```python
from build123d import *

# Parameters (mm, degrees)
SKETCH_1_R          = 1.6
EXTRUDE_1_DEPTH     = 3
SKETCH_2_W          = 11
SKETCH_2_H          = 38
CUT_EXTRUDE_1_DEPTH = 1
CUT_EXTRUDE_START   = -2
CUT_EXTRUDE_2_DEPTH = 2
SKETCH_4_R          = 1.6
CUT_EXTRUDE_3_DEPTH = 62.990079852
SKETCH_6_R          = 2
CUT_EXTRUDE_4_DEPTH = 1
SKETCH_7_R          = 4.1
CUT_EXTRUDE_5_DEPTH = 63.030395775
FILLET_1_R          = 1


with BuildPart() as part:
    # 草图1 → 凸台-拉伸1 (new body)
    with BuildSketch(Plane.XY):
        with BuildLine():
            Line((47.4, -34.9), (47.4, 34.9))
            ThreePointArc((47.4, 34.9), (45.935533906, 38.435533906), (42.4, 39.9))
            Line((42.4, 39.9), (21.6, 39.9))
            ThreePointArc((21.6, 39.9), (18.064466094, 38.435533906), (16.6, 34.9))
            Line((16.6, 34.9), (16.6, -34.9))
            ThreePointArc((16.6, -34.9), (18.064466094, -38.435533906), (21.6, -39.9))
            Line((21.6, -39.9), (42.4, -39.9))
            ThreePointArc((42.4, -39.9), (45.935533906, -38.435533906), (47.4, -34.9))
        make_face()
        with Locations((37.413843028, 25.79305128)):
            Circle(SKETCH_1_R, mode=Mode.SUBTRACT)
        with Locations((31.413843028, 25.79305128)):
            Circle(SKETCH_1_R, mode=Mode.SUBTRACT)
        with BuildLine():
            Line((40.513850359, -21.477641558), (40.513850359, -10.127641653))
            ThreePointArc((40.513850359, -10.127641653), (40.367403749, -9.774088262), (40.013850359, -9.627641653))
            Line((40.013850359, -9.627641653), (30.013850359, -9.627641653))
            ThreePointArc((30.013850359, -9.627641653), (29.660296968, -9.774088262), (29.513850359, -10.127641653))
            Line((29.513850359, -10.127641653), (29.513850359, -21.477641558))
            ThreePointArc((29.513850359, -21.477641558), (29.660296968, -21.831194949), (30.013850359, -21.977641558))
            Line((30.013850359, -21.977641558), (40.013850359, -21.977641558))
            ThreePointArc((40.013850359, -21.977641558), (40.367403749, -21.831194949), (40.513850359, -21.477641558))
        make_face(mode=Mode.SUBTRACT)
        with BuildLine():
            Line((40.464996896, 6.495389649), (40.464996896, -6.604609867))
            ThreePointArc((40.464996896, -6.604609867), (40.406418252, -6.746031223), (40.264996896, -6.804609867))
            Line((40.264996896, -6.804609867), (28.963873947, -6.804609867))
            ThreePointArc((28.963873947, -6.804609867), (28.822452591, -6.746031223), (28.763873947, -6.604609867))
            Line((28.763873947, -6.604609867), (28.763873947, 6.495389649))
            ThreePointArc((28.763873947, 6.495389649), (28.822452591, 6.636811005), (28.963873947, 6.695389649))
            Line((28.963873947, 6.695389649), (40.264996896, 6.695389649))
            ThreePointArc((40.264996896, 6.695389649), (40.406418252, 6.636811005), (40.464996896, 6.495389649))
        make_face(mode=Mode.SUBTRACT)
        with BuildLine():
            Line((40.513843009, 11.302412116), (40.513843009, 19.702429875))
            ThreePointArc((40.513843009, 19.702429875), (40.396685721, 19.985272588), (40.113843009, 20.102429875))
            Line((40.113843009, 20.102429875), (29.713821303, 20.102429875))
            ThreePointArc((29.713821303, 20.102429875), (29.43097859, 19.985272588), (29.313821303, 19.702429875))
            Line((29.313821303, 19.702429875), (29.313821303, 11.302412116))
            ThreePointArc((29.313821303, 11.302412116), (29.43097859, 11.019569403), (29.713821303, 10.902412116))
            Line((29.713821303, 10.902412116), (40.113843009, 10.902412116))
            ThreePointArc((40.113843009, 10.902412116), (40.396685721, 11.019569403), (40.513843009, 11.302412116))
        make_face(mode=Mode.SUBTRACT)
    extrude(amount=-EXTRUDE_1_DEPTH)

    # 草图2 → 切除-拉伸1 (cut)
    with BuildSketch(Plane(origin=(0, 0, -3), x_dir=(-1, 0, 0), z_dir=(0, 0, -1))):
        with Locations((-22.1, 0)):
            Rectangle(SKETCH_2_W, SKETCH_2_H)
    extrude(amount=-CUT_EXTRUDE_1_DEPTH, mode=Mode.SUBTRACT)

    # 草图3 → 切除-拉伸2 (cut)
    with BuildSketch(Plane(origin=(0, 0, -3), x_dir=(-1, 0, 0), z_dir=(0, 0, -1)).offset(CUT_EXTRUDE_START)):
        with BuildLine():
            Line((-47.4, -31.4), (-38.9, -31.4))
            Line((-38.9, -31.4), (-38.9, -39.9))
            Line((-38.9, -39.9), (-42.4, -39.9))
            ThreePointArc((-42.4, -39.9), (-45.935533906, -38.435533906), (-47.4, -34.9))
            Line((-47.4, -34.9), (-47.4, -31.4))
        make_face()
        with BuildLine():
            Line((-47.4, 34.9), (-47.4, 31.4))
            Line((-47.4, 31.4), (-38.9, 31.4))
            Line((-38.9, 31.4), (-38.9, 39.9))
            Line((-38.9, 39.9), (-42.4, 39.9))
            ThreePointArc((-42.4, 39.9), (-45.935533906, 38.435533906), (-47.4, 34.9))
        make_face()
        with BuildLine():
            Line((-16.6, 31.4), (-25.1, 31.4))
            Line((-25.1, 31.4), (-25.1, 39.9))
            Line((-25.1, 39.9), (-21.6, 39.9))
            ThreePointArc((-21.6, 39.9), (-18.064466094, 38.435533906), (-16.6, 34.9))
            Line((-16.6, 34.9), (-16.6, 31.4))
        make_face()
        with BuildLine():
            Line((-16.6, -34.9), (-16.6, -31.4))
            Line((-16.6, -31.4), (-25.1, -31.4))
            Line((-25.1, -31.4), (-25.1, -39.9))
            Line((-25.1, -39.9), (-21.6, -39.9))
            ThreePointArc((-21.6, -39.9), (-18.064466094, -38.435533906), (-16.6, -34.9))
        make_face()
    extrude(amount=CUT_EXTRUDE_2_DEPTH, mode=Mode.SUBTRACT)

    # 草图4 → 切除-拉伸3 (cut, through all)
    with BuildSketch(Plane(origin=(0, 0, -1), x_dir=(-1, 0, 0), z_dir=(0, 0, -1))):
        with Locations((-20.872307757, 35.627692243)):
            Circle(SKETCH_4_R)
        with Locations(Location((-20.872307757, -35.627692243, 0), (0, 0, 180))):
            Circle(SKETCH_4_R)
        with Locations((-43.127692243, -35.627692243)):
            Circle(SKETCH_4_R)
        with Locations(Location((-43.127692243, 35.627692243, 0), (0, 0, 180))):
            Circle(SKETCH_4_R)
    extrude(amount=-CUT_EXTRUDE_3_DEPTH, mode=Mode.SUBTRACT)

    # 草图6 → 切除-拉伸4 (cut)
    with BuildSketch(Plane(origin=(0, 0, -3), x_dir=(-1, 0, 0), z_dir=(0, 0, -1))):
        with Locations((-37.413843028, 25.79305128)):
            Circle(SKETCH_6_R)
        with Locations((-31.413843028, 25.79305128)):
            Circle(SKETCH_6_R)
    extrude(amount=-CUT_EXTRUDE_4_DEPTH, mode=Mode.SUBTRACT)

    # 草图7 → 切除-拉伸5 (cut, through all)
    with BuildSketch(Plane.XY):
        with Locations((32, -30.938820779)):
            Circle(SKETCH_7_R)
    extrude(amount=-CUT_EXTRUDE_5_DEPTH, mode=Mode.SUBTRACT)

    # 圆角1
    fillet_1_edges = [part.edges().sort_by_distance(p)[0] for p in [
        (25.1, -39.9, -2),
        (16.6, -31.4, -2),
        (16.6, 31.4, -2),
        (25.1, 39.9, -2),
        (38.9, 39.9, -2),
        (47.4, 31.4, -2),
        (47.4, -31.4, -2),
        (38.9, -39.9, -2),
    ]]
    fillet(fillet_1_edges, radius=FILLET_1_R)


solid = part.part
```
Model file for the job. Use its own axes, mm. A direction names the side the tool comes from. Coordinates: 2 decimals unless noted, no trailing zeros. Order: outer loops, then holes, each group sorted by start corner. A loop starts at its lowest first (then second) coordinate and runs counter-clockwise, first axis right, second up. Notation, with made-up numbers: (45.5, 41.25) - (72.5, 41.25) arc R16 ccw to (72.5, 62.25) - close; hole circle Ø9 at (82, -37). An arc over 180 degrees is marked (long way). Return JSON: item names as keys, results as strings. Group by question number.
1) Saw through at C-C, the plane y = -8. Write the cut outline in (x, z).
2) Saw through at B-B, the plane x = 44. Write the cut outline in (y, z).
3) Saw through at A-A, the plane y = -17. Write the cut outline in (x, z).
4) Probe line 1 (X direction, y = -12.5, z = -2.65); line 2 (X direction, y = -21.5, z = -1); line 3 (Y direction, x = 37, z = -1.7). List the from-to ranges inside material, lowest first. Write a range as from..to.
5) Tool access for faces 4 (the flat face through (25.1, -35, -2)), 5 (the flat face through (40.514, 15, -1)), 6 (the flat face through (25.1, 35, -2)), 7 (the flat face through (38.9, -35, -2)), 8 (the flat face through (33, 25, -2)): list every direction of +Z, -Z, +X, -X, +Y, -Y with a clear straight run to the whole face (end or side of a thin tool).
6) Mould opens along X. For faces 1 (the cylindrical face through (18.1, 38.47, -0.49)), 2 (the flat face through (47.4, 0, -1)), 3 (the flat face through (29.314, 16, -1)) say: released by +X, released by -X, zero draft, split by the parting line, or undercut.
7) Saw through at D-D, the plane x = 32. Write the cut outline in (y, z).
8) Flat gauge pins, fed straight in: P1, Ø0.5, axis at x = 22.5, z = -2.5, coming from the +Y side; P2, Ø4, axis at x = 43.13, y = 35.63, coming from the -Z side. Where does each tip first touch, or does it go through?
Values found:
{
 "1": {"outline": "(16.6, -2) - (27.6, -2) - (27.6, -3) - (47.4, -3) - (47.4, 0) - (16.6, 0) - close"},
 "2": {"outline": "(-39.64, -1) - (-36.97, -1) - (-36.97, 0) - (-39.64, 0) - close; (-34.29, -1) - (-31.4, -1) - (-31.4, -3) - (31.4, -3) - (31.4, -1) - (34.29, -1) - (34.29, 0) - (-34.29, 0) - close; (36.97, -1) - (39.64, -1) - (39.64, 0) - (36.97, 0) - close"},
 "3": {"outline": "(16.6, -2) - (27.6, -2) - (27.6, -3) - (29.51, -3) - (29.51, 0) - (16.6, 0) - close; (40.51, -3) - (47.4, -3) - (47.4, 0) - (40.51, 0) - close"},
 "4": {"line 1": "x = 27.6..29.51, 40.51..47.4", "line 2": "x = 16.6..29.51, 40.51..47.4", "line 3": "y = -39.9..-21.98, -9.63..-6.8, 6.7..10.9, 20.1..24.25, 27.34..39.9"},
 "5": {"face 4": "-Z, -X, -Y", "face 5": "+Z, -Z", "face 6": "-Z, -X, +Y", "face 7": "-Z, +X, -Y", "face 8": "-Z"},
 "6": {"face 1": "released by -X", "face 2": "released by +X", "face 3": "undercut"},
 "7": {"outline": "(-39.9, -3) - (-35.04, -3) - (-35.04, 0) - (-39.9, 0) - close; (-26.84, -3) - (-21.98, -3) - (-21.98, 0) - (-26.84, 0) - close; (-9.63, -3) - (-6.8, -3) - (-6.8, 0) - (-9.63, 0) - close; (6.7, -3) - (10.9, -3) - (10.9, 0) - (6.7, 0) - close; (20.1, -3) - (23.88, -3) - (23.88, -2) - (24.3, -2) - (24.3, 0) - (20.1, 0) - close; (27.28, -2) - (27.71, -2) - (27.71, -3) - (39.9, -3) - (39.9, 0) - (27.28, 0) - close"},
 "8": {"P1": "stops at y = 31.4", "P2": "stops at z = -1"}
}
